```python
from build123d import *

# Parameters (mm, degrees)
SKETCH2_OUTSIDE_W  = 66.612
SKETCH2_OUTSIDE_H  = 66.612
CUT_EXTRUDE1_DEPTH = 15.2748
FILLET1_R          = 0.381


with BuildPart() as part:
    # Sketch1 → Revolve1 (revolve)
    with BuildSketch(Plane(origin=(0, 0, 0), x_dir=(0, 0, -1), z_dir=(1, 0, 0)), mode=Mode.PRIVATE) as revolve1_sk:
        with BuildLine():
            Line((0, 24.792737963), (0, 6.477))
            Line((0, 6.477), (-3.175, 6.477))
            Line((-3.175, 6.477), (-4.5212, 7.8232))
            Line((-4.5212, 7.8232), (-11.3538, 7.8232))
            Line((-11.3538, 7.8232), (-12.7, 6.477))
            Line((-12.7, 6.477), (-12.7, 0))
            Line((-12.7, 0), (14.2748, 0))
            ThreePointArc((14.2748, 0), (14.26614516, 0.065740037), (14.240770453, 0.127))
            Line((14.240770453, 0.127), (0, 24.792737963))
        make_face()
    revolve(revolve1_sk.sketch.rotate(Axis((0, 0, 0), (0, 0, 1)), 90), axis=Axis((0, 0, 0), (0, 0, 1)))  # turned: the seam where the file's is

    # Sketch2 outside → Cut-Extrude1 (cut, through all)
    with BuildSketch(Plane.XY):
        Rectangle(SKETCH2_OUTSIDE_W, SKETCH2_OUTSIDE_H)
        Polygon((0, 14.664696837), (-12.7, 7.332348419), (-12.7, -7.332348419), (0, -14.664696837), (12.7, -7.332348419), (12.7, 7.332348419), align=None, mode=Mode.SUBTRACT)
    extrude(amount=-CUT_EXTRUDE1_DEPTH, mode=Mode.SUBTRACT)

    # Fillet1
    fillet1_edges = [part.edges().sort_by_distance(p)[0] for p in [
        (6.477, 0, 0),
    ]]
    fillet(fillet1_edges, radius=FILLET1_R)


solid = part.part
```
Verification items for the finished model (mm, model axes). A direction names the side the tool comes from. Give positions to 0.01 mm unless a question says otherwise; leave off trailing zeros. Order: outer loops, then holes, each group sorted by start corner. A loop starts at its lowest first (then second) coordinate and runs counter-clockwise, first axis right, second up. Notation, with made-up numbers: M -0.5,-18.75 L 14.5,-18.75 A26 ccw 14.5,-0.75 Z; hole C 69,-18 d8. An arc over 180 degrees is marked long. Return JSON: item names as keys, results as strings. Group by question number.
1) Go/stop test with flat-tipped pins: pin 1 Ø6 at (y, z) = (1, 10) entering from +X; pin 2 Ø4 at (x, z) = (8, -0.5) entering from +Y; pin 3 Ø4 at (x, y) = (7.5, 5.5) entering from -Z. Record where each tip stops, or that it passes through.
2) Mould release check, pull along Z, two halves, no side actions. Record for faces 1 (the face through (-12.7, 0, -3)), 2 (the face through (1.404, 6.323, 1.798)), 3 (the face through (-0.989, -0.311, -13.716)): pulls with the +Z half, pulls with the -Z half, needs draft (parallel to the pull), parting line crosses it, or undercut.
3) Section check B-B on z = 7.75. Record the cut outline in (x, y).
4) Scan lines: line 1 (Z direction, x = 10.5, y = 4); line 2 (Y direction, x = 2, z = -4); line 3 (X direction, y = -3, z = -7.75). Record each from-to range of solid material in increasing order.
5) Access from +Z, -Z, +X, -X, +Y, -Y to the whole of each face (thin tool, end or side, straight path). Record for faces 4 (the face through (-7.46, -2.35, 7.99)), 5 (the face through (6.26, -11.05, -3.44)).
6) Section check A-A on z = -0.5. Record the cut outline in (x, y).
7) Section check C-C on z = -7.5. Record the cut outline in (x, y).
Answer block:
{
 "1": {"pin 1": "stops at x = 7.82", "pin 2": "stops at y = 11.2", "pin 3": "stops at z = -10.1"},
 "2": {"face 1": "needs draft", "face 2": "undercut", "face 3": "pulls with the -Z half"},
 "3": {"outline": "C 0,0 d15.65"},
 "4": {"line 1": "z = -7.83 to 0", "line 2": "y = -13.51 to 13.51", "line 3": "x = -10.97 to 10.97"},
 "5": {"face 4": "+Z", "face 5": "+Z, -Z, +X, -Y"},
 "6": {"outline": "M -12.7,-7.33 L 0,-14.66 L 12.7,-7.33 L 12.7,7.33 L 0,14.66 L -12.7,7.33 Z"},
 "7": {"outline": "C 0,0 d23.6"}
}
